Check sheet for the modelled part. Datum: model origin and axes. Units: mm. A direction names the side the tool comes from. Round coordinates to 2 decimals unless told otherwise and drop trailing zeros. Write each loop counter-clockwise with the first axis right and the second up, starting at its lowest first coordinate (ties: lowest second). Pieces come first, ordered by that corner, then holes. Notation, with made-up numbers: (84.25, 44.25) -> (100.25, 44.25) arc R20 ccw to (100.25, 75.25) -> close; hole circle Ø3 at (50, -33). An arc over 180 degrees is marked (long way). One line per item, written item: value.
from build123d import *

# Parameters (mm, degrees)
BOSS_EXTRUDE1_DEPTH      = 50
SHELL1_T                 = -5
BOSS_EXTRUDE2_DEPTH      = 5.500000000000001
BOSS_EXTRUDE2_DEPTH_BACK = 7.5
CUT_EXTRUDE1_DEPTH       = 10
SKETCH5_W                = 16
SKETCH5_H                = 5
CUT_EXTRUDE2_DEPTH       = 121.69448930041943
FILLET2_RADIUS           = 2.5
FILLET2_LENGTH           = 40
FILLET3_RADIUS           = 2.5
FILLET3_LENGTH           = 40


with BuildPart() as part:
    # Sketch2 → Boss-Extrude1 (new body)
    with BuildSketch(Plane(origin=(0, 0, 0), x_dir=(1, 0, 0), z_dir=(0, 1, 0))):
        with BuildLine():
            Line((18.78053977456615, -77.31409286467196), (23.042995642351375, -79.77502290734665))
            Line((23.042995642351375, -79.77502290734665), (31.523043656078794, -84.67098091081314))
            Line((31.523043656078794, -84.67098091081314), (31.773043656078798, -84.23796820892092))
            Line((31.773043656078798, -84.23796820892092), (45.62945011662982, -92.23796820892092))
            Line((45.62945011662982, -92.23796820892092), (72.62945011662983, -45.4725964045612))
            Line((72.62945011662983, -45.4725964045612), (58.773043656078805, -37.472596404561216))
            Line((58.773043656078805, -37.472596404561216), (59.0230436560788, -37.039583702669006))
            Line((59.0230436560788, -37.039583702669006), (50.362789618234416, -32.03958370266901))
            Line((50.362789618234416, -32.03958370266901), (46.10033375044919, -29.578653659994334))
            add(Edge.make_bspline(
                [(18.78053977456615, -77.31409286467196), (38.540581097928744, -63.49650278099066), (46.10033375044919, -29.578653659994334)],
                knots=[3.5325222979989195, 3.5325222979989195, 3.5325222979989195, 4.350849853477907, 4.350849853477907, 4.350849853477907], degree=2, weights=[1, 0.9174538281146124, 1]))
        make_face()
    extrude(amount=BOSS_EXTRUDE1_DEPTH)

    # Shell1
    shell1_openings = [part.faces().sort_by_distance(p)[0] for p in [
        (47.213884273, 50, 61.782899624),
        (47.213884273, 0, 61.782899624),
        (59.129450117, 25, 68.855282307),
    ]]
    offset(amount=SHELL1_T, openings=shell1_openings, kind=Kind.INTERSECTION)

    # Sketch3 → Boss-Extrude2 (add, two sides: drawn at the far end of the back side and taken through both)
    with BuildSketch(Plane(origin=(47.47757848615084, 0, 27.172215953725974), x_dir=(-0.4967199718961618, 0, 0.8679108649622244), z_dir=(-0.8679108649622244, 0, -0.4967199718961618)).offset(-BOSS_EXTRUDE2_DEPTH_BACK)):
        Polygon((25.664850284699074, 37.339555568810255), (28.453024038902463, 35.000000000000014), (32.09272638156445, 35.000000000000014), (34.8809001357678, 37.339555568810226), (35.51292781482111, 40.92396265452046), (33.69307664349011, 44.07603734547951), (30.272875210233437, 45.320888862379554), (26.852673776976776, 44.07603734547953), (25.03282260564577, 40.923962654520494), align=None)
        Polygon((33.69307664349011, 5.923962654520468), (35.51292781482114, 9.07603734547954), (34.880900135767824, 12.660444431189784), (32.09272638156446, 15.000000000000004), (28.453024038902413, 15.000000000000004), (25.664850284699046, 12.660444431189786), (25.032822605645727, 9.07603734547953), (26.852673776976744, 5.9239626545204755), (30.272875210233433, 4.679111137620436), align=None)
    extrude(amount=BOSS_EXTRUDE2_DEPTH + BOSS_EXTRUDE2_DEPTH_BACK)

    # Sketch4 → Cut-Extrude1 (cut)
    with BuildSketch(Plane(origin=(47.47757848615084, 0, 27.172215953725974), x_dir=(-0.4967199718961618, 0, 0.8679108649622244), z_dir=(-0.8679108649622244, 0, -0.4967199718961618))):
        Polygon((40.272875210233444, 19.999999999999996), (20.27287521023344, 19.999999999999993), (20.27287521023344, 30), (40.272875210233444, 30.000000000000007), align=None)
    extrude(amount=-CUT_EXTRUDE1_DEPTH, mode=Mode.SUBTRACT)

    # Sketch5 → Cut-Extrude2 (cut, through all)
    with BuildSketch(Plane(origin=(-28.532849302036027, 0, 49.420344675832624), x_dir=(0.8660254037844389, 0, 0.49999999999999967), z_dir=(-0.49999999999999967, 0, 0.8660254037844389))):
        with Locations((77.63524706617667, 47.50000000000001)):
            Rectangle(SKETCH5_W, SKETCH5_H)
        Polygon((69.63524706617666, 0), (85.63524706617667, 0), (85.63524706617667, 5), (69.63524706617667, 4.999999999999997), align=None)
    extrude(amount=-CUT_EXTRUDE2_DEPTH, mode=Mode.SUBTRACT)

    # Fillet2: full round fillet: the end face becomes a half cylinder, R = half its width
    fillet2_face = Plane((46.879450117, 25, 90.072904699), x_dir=(0, 1, 0), z_dir=(0.866025403784, 0, 0.5))  # on the end face: x along it, z out of the body
    fillet2_slab = fillet2_face.offset(-FILLET2_RADIUS / 2) * Box(FILLET2_LENGTH, 2 * FILLET2_RADIUS, FILLET2_RADIUS, mode=Mode.PRIVATE)  # the body's end, R deep
    fillet2_round = Plane((44.71438660754, 25, 88.822904699), x_dir=(0.866025403784, 0, 0.5), z_dir=(0, 1, 0)) * Cylinder(FILLET2_RADIUS, FILLET2_LENGTH, mode=Mode.PRIVATE)  # its axis R under the face
    add(fillet2_slab - fillet2_round, mode=Mode.SUBTRACT)

    # Fillet3: full round fillet: the end face becomes a half cylinder, R = half its width
    fillet3_face = Plane((71.379450117, 25, 47.637659914), x_dir=(0, -1, 0), z_dir=(0.866025403784, 0, 0.5))  # on the end face: x along it, z out of the body
    fillet3_slab = fillet3_face.offset(-FILLET3_RADIUS / 2) * Box(FILLET3_LENGTH, 2 * FILLET3_RADIUS, FILLET3_RADIUS, mode=Mode.PRIVATE)  # the body's end, R deep
    fillet3_round = Plane((69.21438660754, 25, 46.387659914), x_dir=(0.866025403784, 0, 0.5), z_dir=(0, -1, 0)) * Cylinder(FILLET3_RADIUS, FILLET3_LENGTH, mode=Mode.PRIVATE)  # its axis R under the face
    add(fillet3_slab - fillet3_round, mode=Mode.SUBTRACT)


solid = part.part
Item 1: Depth check by flat-ended pin: P1, Ø5, axis at x = 51, y = 36, coming from the +Z side; P2, Ø5, axis at x = 51.5, y = 33, coming from the -Z side; P3, Ø9, axis at x = 39.5, z = 83, coming from the -Y side. Enter the tip coordinate at first touch or a pass-through.
Answer:
P1: stops at z = 40.2
P2: stops at z = 31.25
P3: stops at y = 5
Item 2: Thickness scan on line 1 (X direction, y = 29, z = 40.5); line 2 (Z direction, x = 26, y = 43.5); line 3 (Z direction, x = 35, y = 29.5). Record the ranges inside material, lowest first.
Answer:
line 1: x = 43.12 to 48.37, 54.02 to 64.02
line 2: z = 53.63 to 54.08, 71.04 to 81.48
line 3: z = 66.43 to 68.01, 80.33 to 86.1
Item 3: Tool access check on faces 4 (the flat face through (28.593, 24.65, 77.206)), 5 (the flat face through (34.56, 39.16, 48.98)), 6 (the flat face through (34.298, 42.522, 49.535)), 7 (the flat face through (29.8, 39.1, 57.6)). Record the directions out of +Z, -Z, +X, -X, +Y, -Y that give a thin tool (end or side, any length) a straight path to the whole face; none if there is none.
Answer:
face 4: +Y, -Y
face 5: -Z
face 6: -Z, +Y
face 7: -X
Item 4: Sectioned sample at A-A on x = 62.5. Enter the section's corners in (y, z), and give its area (3 significant figures).
Answer:
outline: (5, 39.62) -> (45, 39.62) -> (45, 45.4) -> (5, 45.4) -> close
area: 231 mm^2
Item 5: Mould release check, pull along X, two halves, no side actions. Record for faces 1 (the flat face through (65, 5, 44)), 2 (the flat face through (30.11, 7.48, 57.09)), 3 (the flat face through (33.09, 5.31, 51.82)): pulls with the +X half, pulls with the -X half, needs draft (parallel to the pull), parting line crosses it, or undercut.
Answer:
face 1: needs draft
face 2: pulls with the -X half
face 3: undercut
Item 6: Sectioned sample at B-B on x = 54.5. Enter the section's corners in (y, z).
Answer:
outline: (0, 34.43) -> (50, 34.43) -> (50, 40.78) -> (0, 40.78) -> close
